from build123d import *

# Parameters (mm, degrees)
EXTRUDE_THIN1_DEPTH = 539.75
FILLET1_R           = 1.27


with BuildPart() as part:
    # Sketch1 → Extrude-Thin1 (new body)
    with BuildSketch(Plane.XY):
        Polygon((0, 49.2125), (0, 53.975), (-28.575, 53.975), (-28.575, 44.45), (-25.4, 44.45), (-9.525, 7.9375), (-6.35, 7.9375), (-6.35, 0), (0, 0), (0, 4.7625), (-1.27, 4.7625), (-1.27, 1.27), (-5.08, 1.27), (-5.08, 9.2075), (-8.692328784, 9.2075), (-24.567328784, 45.72), (-27.305, 45.72), (-27.305, 52.705), (-1.27, 52.705), (-1.27, 49.2125), align=None)
    extrude(amount=-EXTRUDE_THIN1_DEPTH)

    # Fillet1
    fillet1_edges = [part.edges().sort_by_distance(p)[0] for p in [
        (0, 0, -269.875),
        (-6.35, 0, -269.875),
        (-9.525, 7.9375, -269.875),
        (-28.575, 44.45, -269.875),
        (-28.575, 53.975, -269.875),
        (0, 53.975, -269.875),
        (-24.567328784, 45.72, -269.875),
        (-5.08, 9.2075, -269.875),
    ]]
    fillet(fillet1_edges, radius=FILLET1_R)


solid = part.part
Work out the finished part from the listing and answer in its coordinate system (mm). Give positions to 0.01 mm unless a question says otherwise; leave off trailing zeros. Loops run counter-clockwise (first coordinate to the right, second up) from the corner with the lowest first, then second, coordinate; pieces in that order, holes last. Notation, with made-up numbers: (-27.75, 11) - (-8.75, 11) arc R13 cw to (-8.75, 35) - close; hole circle Ø11 at (-36, 52.5). An arc over 180 degrees is marked (long way). Answer in a Markdown table with one row per item.
(1) Flat-ended cylindrical pins translate along their axes: pin 1 Ø3 at (y, z) = (3.5, -143) entering from -X; pin 2 Ø1 at (x, z) = (-0.5, -335) entering from +Y; pin 3 Ø0.7 at (x, z) = (-7, -270.5) entering from -Y. Find the tip coordinate at first contact, or state that the pin passes through.
Results list:
| item | result |
|---|---|
| pin 1 | stops at x = -6.35 |
| pin 2 | stops at y = 53.95 |
| pin 3 | stops at y = 7.94 |
(2) Section C-C (y = 19) is taken. Give the vertices of the cut face in (x, z).
Results list:
| item | result |
|---|---|
| outline | (-14.33, -539.75) - (-12.95, -539.75) - (-12.95, 0) - (-14.33, 0) - close |
(3) Consider L1, parallel to Y at x = -8, z = -374.5 (1 decimal); L2, parallel to Y at x = -22.5, z = -266 (3 decimals); L3, parallel to X at y = 5, z = -332. Determine where each line is inside the solid, lowest interval first. Write a range as [from, to].
Results list:
| item | result |
|---|---|
| L1 | y = [7.9, 9.2], [52.7, 54] |
| L2 | y = [37.78, 40.965], [52.705, 53.975] |
| L3 | x = [-6.35, -5.08] |
(4) For a pull along X with two mould halves and no side action, classify faces 1 (the face through (-14, 53.975, -266)), 2 (the face through (-16.355, 26.832, -266.097)), 3 (the face through (-14, 52.705, -266)), 4 (the face through (-17.74, 26.83, -266.1)) as pulls with the +X half, pulls with the -X half, needs draft (parallel to the pull), parting line crosses it, or undercut.
Results list:
| item | result |
|---|---|
| face 1 | needs draft |
| face 2 | pulls with the +X half |
| face 3 | undercut |
| face 4 | pulls with the -X half |
(5) Section A-A (x = -16.75) is taken. Give the vertices of the cut face in (y, z) (3 decimals).
Results list:
| item | result |
|---|---|
| outline | (24.555, -539.75) - (27.74, -539.75) - (27.74, 0) - (24.555, 0) - close; (52.705, -539.75) - (53.975, -539.75) - (53.975, 0) - (52.705, 0) - close |
